The drawing under review shows one solid part. Ordinate dimensions are in mm from its lowest x, y, z. A direction names the side the tool comes from. Coordinates: 2 decimals unless noted, no trailing zeros. Write each loop counter-clockwise with the first axis right and the second up, starting at its lowest first coordinate (ties: lowest second). Pieces come first, ordered by that corner, then holes. Notation, with made-up numbers: (82, 46.5) - (137, 46.5) arc R14 cw to (137, 51.5) - close; hole circle Ø4 at (6.5, 70). An arc over 180 degrees is marked (long way). Put each result on its own line as item: value. Start each with the question number.
Item 1: To check wall thickness, follow L1, parallel to Y at x = 28, z = 6.5 (1 decimal); L2, parallel to Y at x = 21, z = 25.5 (1 decimal); L3, parallel to X at y = 3, z = 17. State the ranges of each line that lie inside material, in increasing order. Write a range as [from, to].
Item 2: Mouldability with a two-part tool opening along Y and no side actions: class the marked faces 3, 4, 5 and 6 as pulls with the +Y half, pulls with the -Y half, needs draft (parallel to the pull), parting line crosses it, or undercut.
Item 3: Machinability: for the marked faces 1 and 2, which of the approach directions +Z, -Z, +X, -X, +Y, -Y give a long, thin tool a straight path to every point of the face, cutting with its end or side? Answer none if there is none.
Item 4: Consider section C-C on z = 17.5. Give the boundary of the cut face in (x, y) (1 decimal).
Item 5: Consider section B-B on z = 9. Give the boundary of the cut face in (x, y) (1 decimal).
Item 6: For pin 1 (3 mm diameter, centred on x = 13, z = 4.5, fed in from -Y); pin 2 (0.5 mm diameter, centred on y = 0.5, z = 10.5, fed in from -X); pin 3 (11.5 mm diameter, centred on x = 14.29, z = 15.88, fed in from +Y) (1 decimal); pin 4 (3 mm diameter, centred on y = 10.5, z = 15, fed in from -X), all flat-tipped, find the tip position at first contact; note any pin that passes through.
Item 7: Consider section D-D on y = 5.5. Give the boundary of the cut face in (x, z).
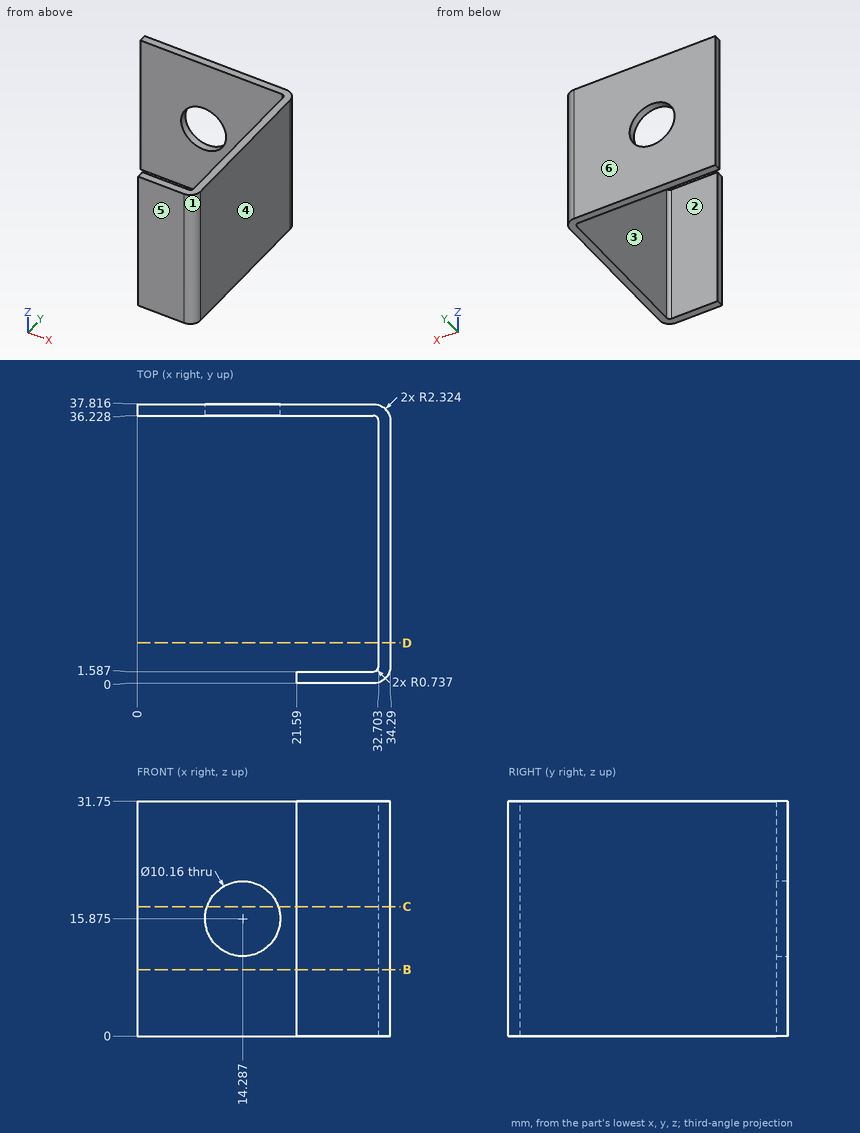
Report:
1. L1: [0, 1.6], [36.2, 37.8]
1. L2: [36.2, 37.8]
1. L3: [32.7, 34.29]
2. face 3: undercut
2. face 4: needs draft
2. face 5: pulls with the -Y half
2. face 6: pulls with the +Y half
3. face 1: +Z, -Z, +X, -Y
3. face 2: +Z, -Z, -X
4. outline: (0, 36.2) - (9.5, 36.2) - (9.5, 37.8) - (0, 37.8) - close; (19.1, 36.2) - (32, 36.2) arc R0.7 cw to (32.7, 35.5) - (32.7, 2.3) arc R0.7 cw to (32, 1.6) - (21.6, 1.6) - (21.6, 0) - (32, 0) arc R2.3 ccw to (34.3, 2.3) - (34.3, 35.5) arc R2.3 ccw to (32, 37.8) - (19.1, 37.8) - close
5. outline: (0, 36.2) - (32, 36.2) arc R0.7 cw to (32.7, 35.5) - (32.7, 2.3) arc R0.7 cw to (32, 1.6) - (21.6, 1.6) - (21.6, 0) - (32, 0) arc R2.3 ccw to (34.3, 2.3) - (34.3, 35.5) arc R2.3 ccw to (32, 37.8) - (0, 37.8) - close
6. pin 1: y = 36.23
6. pin 2: x = 21.59
6. pin 3: y = 37.8
6. pin 4: x = 32.7
7. outline: (32.7, 0) - (34.29, 0) - (34.29, 31.75) - (32.7, 31.75) - close
